```python
from build123d import *

# Parameters (mm, degrees)
F4_W     = 3
F4_H     = 9
F5_DEPTH = 25


with BuildPart() as f3:
    # F0 (on Top) → F3 section 0
    with BuildSketch(Plane.XY):
        Polygon((-66.641917, 50.499433), (-56.641917, 50.499433), (3.358083, 50.499433), (3.358083, -117.500567), (36.858083, -117.500567), (36.858083, -77.500567), (28.858083, -77.500567), (28.858083, -111.500567), (8.358083, -111.500567), (8.358083, 63.499433), (-66.641917, 63.499433), align=None)
    # F2 (on offset) → F3 section 1
    with BuildSketch(Plane.XY.offset(19)):
        Polygon((-71.641917, 50.499433), (-61.641917, 50.499433), (-1.641917, 50.499433), (-1.641917, -117.500567), (31.858083, -117.500567), (31.858083, -77.500567), (23.858083, -77.500567), (23.858083, -111.500567), (3.358083, -111.500567), (3.358083, 63.499433), (-71.641917, 63.499433), align=None)
    loft()

    # F4 (on face) → F5 (cut)
    with BuildSketch(Plane.XY.offset(19)):
        with Locations((-62.141917, 54.999433)):
            Rectangle(F4_W, F4_H)
    extrude(amount=-F5_DEPTH, mode=Mode.SUBTRACT)


solid = f3.part
```
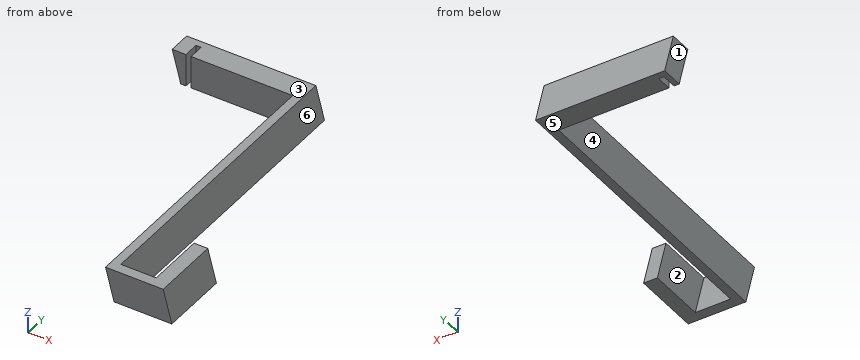
Input: part model. Units: mm. Frame: model coordinates. Face numbers are marked on the shaded views. A direction names the side the tool comes from. Give positions to 0.01 mm unless a question says otherwise; leave off trailing zeros. Order: outer loops, then holes, each group sorted by start corner. A loop starts at its lowest first (then second) coordinate and runs counter-clockwise, first axis right, second up. Notation, with made-up numbers: M -27,16.25 L 18,16.25 A9 ccw 18,22.25 Z; hole C 54.5,44 d6. An arc over 180 degrees is marked long. Return JSON: item names as keys, results as strings.
Item 1: Cut plane A-A (y = -99). Return loops of the section in (x, z), then the cut area to 3 significant figures.
Solutions:
{"outline": "M -1.64,19 L 3.36,0 L 8.36,0 L 3.36,19 Z; M 23.86,19 L 28.86,0 L 36.86,0 L 31.86,19 Z", "area": "247 mm^2"}
Item 2: Pull-direction query (X, two-part tool) for the marked faces 1, 2 and 3; classes: +X half, -X half, draft (parallel to the pull), parting line (faces both ways), or undercut.
Solutions:
{"face 1": "-X half", "face 2": "undercut", "face 3": "draft"}
Item 3: Ray query, probe 1 along Y at (x, z) = (-14, 4); probe 2 along X at (y, z) = (-88, 9.5); probe 3 along X at (y, z) = (-90, 17). Return the intervals inside material, ascending.
Solutions:
{"probe 1": "50.5 to 63.5", "probe 2": "0.86 to 5.86, 26.36 to 34.36", "probe 3": "-1.12 to 3.88, 24.38 to 32.38"}
Item 4: First-contact query: P1, Ø2.5, axis at y = 55, z = 9.5, coming from the -X side; P2, Ø0.9, axis at x = -62.5, z = 10.5, coming from the -Y side; P3, Ø7, axis at y = 54, z = 10.5, coming from the +X side. Flat tips, straight axial feed; report the tip coordinate or a pass-through.
Solutions:
{"P1": "x = -69.47", "P2": "y = 59.5", "P3": "x = 6.52"}
Item 5: Cut plane B-B (y = -11.5). Return loops of the section in (x, z), then the cut area to 3 significant figures.
Solutions:
{"outline": "M -1.64,19 L 3.36,0 L 8.36,0 L 3.36,19 Z", "area": "95.0 mm^2"}
Item 6: Access query for the marked faces 4, 5 and 6. Directions: +Z, -Z, +X, -X, +Y, -Y. A direction counts if a zero-diameter tool reaches every point of the face in a straight line with its end or side. Return the directions, or none.
Solutions:
{"face 4": "-Z, -X, -Y", "face 5": "-Z, +X, -X, +Y, -Y", "face 6": "+Z, +Y"}
